```python
from build123d import *

# Parameters (mm, degrees)
SKETCH3_R               = 8.99487737
SKETCH3_R_2             = 5.99487737
BOSS_EXTRUDE4_DEPTH     = 10
BOSS_EXTRUDE5_START     = 15
SKETCH4_R               = 12.45
BOSS_EXTRUDE5_DEPTH     = 15
CUT_EXTRUDE1_DEPTH      = 37.727817928
CUT_EXTRUDE1_DEPTH_BACK = 37.727817928
SKETCH5_R               = 5


with BuildPart() as part:
    # Sketch2 → Revolve1 (revolve)
    with BuildSketch(Plane(origin=(0, 0, 0), x_dir=(0, 0, -1), z_dir=(1, 0, 0)), mode=Mode.PRIVATE) as revolve1_sk:
        Polygon((0, 0), (0, 12.45), (-5, 12.45), (-5, 10.32), (-7.6162, 10.32), (-7.6162, 12.45), (-9.6162, 12.45), (-9.6162, 10.32), (-12.2324, 10.32), (-12.2324, 12.45), (-17.2324, 12.45), (-17.2324, 0), align=None)
    revolve(revolve1_sk.sketch.rotate(Axis((0, 0, 17.2324), (0, 0, -1)), 180), axis=Axis((0, 0, 17.2324), (0, 0, -1)))

    # Sketch3 → Boss-Extrude4 (add)
    with BuildSketch(Plane(origin=(0, 0, 0), x_dir=(-1, 0, 0), z_dir=(0, 0, -1))):
        with Locations(Location((0, 0, 0), (0, 0, 270))):
            Circle(SKETCH3_R)
        with Locations(Location((0, 0, 0), (0, 0, 90))):
            Circle(SKETCH3_R_2, mode=Mode.SUBTRACT)
    extrude(amount=BOSS_EXTRUDE4_DEPTH)

    # Sketch4 → Boss-Extrude5 (add)
    with BuildSketch(Plane.XY.offset(17.2324).offset(BOSS_EXTRUDE5_START)):
        with Locations(Location((0, 0, 0), (0, 0, 270))):
            Circle(SKETCH4_R)
    extrude(amount=-BOSS_EXTRUDE5_DEPTH)

    # Sketch5 → Cut-Extrude1 (cut, two sides: drawn at the far end of the back side and taken through both)
    with BuildSketch(Plane(origin=(0, 0, 0), x_dir=(0, 0, -1), z_dir=(1, 0, 0)).offset(-CUT_EXTRUDE1_DEPTH_BACK)):
        with Locations((-24.968914218, 0)):
            Circle(SKETCH5_R)
    extrude(amount=CUT_EXTRUDE1_DEPTH + CUT_EXTRUDE1_DEPTH_BACK, mode=Mode.SUBTRACT)


solid = part.part
```
Verification items for the finished model (mm, model axes). A direction names the side the tool comes from. Coordinates: 2 decimals unless noted, no trailing zeros. Loops run counter-clockwise (first coordinate to the right, second up) from the corner with the lowest first, then second, coordinate; pieces in that order, holes last. Notation, with made-up numbers: (-37, 42.25) -> (-26, 42.25) arc R23 ccw to (-26, 51.25) -> close; hole circle Ø9 at (-10, -3). An arc over 180 degrees is marked (long way). Answer in a Markdown table with one row per item. Add a question column.
1. Section check C-C, the plane z = -0.5. Enter the section's corners in (x, y).
2. Material ranges on probe 1 along Z at (x, y) = (-8.25, -6.75); probe 2 along Z at (x, y) = (2.25, 0); probe 3 along Y at (x, z) = (-0.25, 11.5), recorded low to high. Write a range as [from, to].
3. Depth check by flat-ended pin: P1, Ø1, axis at y = -5.5, z = 9.5, coming from the +X side; P2, Ø3.5, axis at x = 3, y = 0, coming from the -Z side; P3, Ø1.5, axis at x = -9, z = 9.5, coming from the -Y side; P4, Ø8, axis at y = 0, z = 24.97, coming from the -X side. Enter the tip coordinate at first touch or a pass-through.
4. Draft check along Y on faces 1 (the face through (-0.174, 0.22, 29.964)), 2 (the face through (11.05, -5.74, 8.63)), 3 (the face through (6, -2, -10)). Enter one of: +Y half, -Y half, draft (parallel to the pull), parting line (faces both ways), or undercut.
5. Access from +Z, -Z, +X, -X, +Y, -Y to the whole of each face (thin tool, end or side, straight path). Record for faces 4 (the face through (6.28, 8.19, 6.33)), 5 (the face through (11.05, -5.74, 2.54)), 6 (the face through (-2.7, -8.58, -4.93)).
6. Section check D-D, the plane x = -7.5. Enter the section's corners in (y, z).
Derived:
| question | item | result |
|---|---|---|
| 1 | outline | circle Ø17.99 at (0, 0); hole circle Ø11.99 at (0, 0) |
| 2 | probe 1 | z = [0, 5], [7.62, 9.62], [12.23, 32.23] |
| 2 | probe 2 | z = [0, 19.97], [29.97, 32.23] |
| 2 | probe 3 | y = [-10.32, 10.32] |
| 3 | P1 | stops at x = 11.4 |
| 3 | P2 | stops at z = 0 |
| 3 | P3 | stops at y = -9.32 |
| 3 | P4 | passes through |
| 4 | face 1 | undercut |
| 4 | face 2 | parting line |
| 4 | face 3 | draft |
| 5 | face 4 | none |
| 5 | face 5 | +Z, -Z |
| 5 | face 6 | -Z |
| 6 | outline | (-9.94, 0) -> (-4.97, 0) -> (-4.97, -10) -> (4.97, -10) -> (4.97, 0) -> (9.94, 0) -> (9.94, 5) -> (7.09, 5) -> (7.09, 7.62) -> (9.94, 7.62) -> (9.94, 9.62) -> (7.09, 9.62) -> (7.09, 12.23) -> (9.94, 12.23) -> (9.94, 32.23) -> (-9.94, 32.23) -> (-9.94, 12.23) -> (-7.09, 12.23) -> (-7.09, 9.62) -> (-9.94, 9.62) -> (-9.94, 7.62) -> (-7.09, 7.62) -> (-7.09, 5) -> (-9.94, 5) -> close; hole circle Ø10 at (0, 24.97) |
